Verification items for the finished model (mm, model axes). A direction names the side the tool comes from. Round coordinates to 2 decimals unless told otherwise and drop trailing zeros. Order: outer loops, then holes, each group sorted by start corner. A loop starts at its lowest first (then second) coordinate and runs counter-clockwise, first axis right, second up. Notation, with made-up numbers: (-35.5, 6) -> (-21.5, 6) arc R16 ccw to (-21.5, 37) -> close; hole circle Ø5 at (17, 32.5). An arc over 180 degrees is marked (long way). Write item = value, one per line. Start each with the question number.
from build123d import *

# Parameters (mm, degrees)
SKETCH1_W            = 208
SKETCH1_H            = 147
BOSS_EXTRUDE1_DEPTH  = 5
CUT_EXTRUDE1_DEPTH   = 129.501744983
SKETCH3_W            = 88.802487793
SKETCH3_H            = 5
CUT_EXTRUDE2_DEPTH   = 5
MIRROR3_COPY_1_DEPTH = 129.501744983
FILLET1_R            = 10
CUT_EXTRUDE3_DEPTH   = 129.501744983
BOSS_EXTRUDE2_DEPTH  = 20
FILLET2_R            = 5
FILLET2_OF_MIRROR4_R = 5
MIRROR5_START        = -20
MIRROR5_DEPTH        = 20


# Read off the part's stored shape, not the designer's step: Mirror5
with BuildPart() as part:
    # Sketch1 → Boss-Extrude1 (new body)
    with BuildSketch(Plane(origin=(0, 0, 0), x_dir=(1, 0, 0), z_dir=(0, 1, 0))):
        with Locations((0, -1.810679612)):
            Rectangle(SKETCH1_W, SKETCH1_H)
    extrude(amount=BOSS_EXTRUDE1_DEPTH)

    # Sketch2 → Cut-Extrude1 (cut, through all)
    with BuildSketch(Plane(origin=(0, 5, 0), x_dir=(1, 0, 0), z_dir=(0, 1, 0))):
        with BuildLine():
            Line((-89, 75), (-89, 55))
            Line((-89, 55), (-44, 55))
            Line((-44, 55), (-44, 50))
            Line((-44, 50), (-29, 50))
            Line((-29, 50), (-29, 53))
            Line((-29, 53), (-14, 53))
            ThreePointArc((-14, 53), (-6.928932188, 53.502525317), (0, 55))
            Line((0, 55), (0, 75))
            Line((0, 75), (-89, 75))
        make_face()
    cut_extrude1 = extrude(amount=-CUT_EXTRUDE1_DEPTH, mode=Mode.SUBTRACT)

    # Mirror1: Cut-Extrude1 across plane
    add(cut_extrude1.mirror(Plane.XY), mode=Mode.SUBTRACT)

    # Sketch3 → Cut-Extrude2 (cut)
    with BuildSketch(Plane.XY.offset(75.310679612)):
        with Locations((-44.401243897, 2.5)):
            Rectangle(SKETCH3_W, SKETCH3_H)
    cut_extrude2 = extrude(amount=-CUT_EXTRUDE2_DEPTH, mode=Mode.SUBTRACT)

    # Mirror3: Cut-Extrude1, Cut-Extrude2 across plane
    add(cut_extrude1.mirror(Plane(origin=(0, 0, 0), x_dir=(0, 0, 1), z_dir=(1, 0, 0))), mode=Mode.SUBTRACT)
    add(cut_extrude2.mirror(Plane(origin=(0, 0, 0), x_dir=(0, 0, 1), z_dir=(1, 0, 0))), mode=Mode.SUBTRACT)

    # Mirror3 copy 1 sketch → Mirror3 copy 1 (cut, through all)
    with BuildSketch(Plane(origin=(0, 5, 0), x_dir=(-1, 0, 0), z_dir=(0, 1, 0))):
        with BuildLine():
            Line((-89, 75), (-89, 55))
            Line((-89, 55), (-44, 55))
            Line((-44, 55), (-44, 50))
            Line((-44, 50), (-29, 50))
            Line((-29, 50), (-29, 53))
            Line((-29, 53), (-14, 53))
            ThreePointArc((-14, 53), (-6.928932188, 53.502525317), (0, 55))
            Line((0, 55), (0, 75))
            Line((0, 75), (-89, 75))
        make_face()
    extrude(amount=-MIRROR3_COPY_1_DEPTH, mode=Mode.SUBTRACT)

    # Fillet1
    fillet1_edges = [part.edges().sort_by_distance(p)[0] for p in [
        (104, 2.5, 75.310679612),
        (-104, 2.5, 75.310679612),
        (-104, 2.5, -71.689320388),
        (104, 2.5, -71.689320388),
    ]]
    fillet(fillet1_edges, radius=FILLET1_R)

    # Sketch4 → Cut-Extrude3 (cut, through all)
    with BuildSketch(Plane(origin=(0, 5, 0), x_dir=(1, 0, 0), z_dir=(0, 1, 0))):
        with BuildLine():
            Line((-52.239573725, -2.137194831), (-52.239573725, -12.224477428))
            ThreePointArc((-52.239573725, -12.224477428), (-52.093127116, -12.578030818), (-51.739573725, -12.724477428))
            Line((-51.739573725, -12.724477428), (-49.914138918, -12.724477428))
            ThreePointArc((-49.914138918, -12.724477428), (-49.560585528, -12.578030818), (-49.414138918, -12.224477428))
            Line((-49.414138918, -12.224477428), (-49.414138918, -2.137194831))
            ThreePointArc((-49.414138918, -2.137194831), (-49.267692309, -1.783641441), (-48.914138918, -1.637194831))
            Line((-48.914138918, -1.637194831), (-37.856129593, -1.637194831))
            ThreePointArc((-37.856129593, -1.637194831), (-37.502576202, -1.490748222), (-37.356129593, -1.137194831))
            Line((-37.356129593, -1.137194831), (-37.356129593, 0.688239976))
            ThreePointArc((-37.356129593, 0.688239976), (-37.502576202, 1.041793366), (-37.856129593, 1.188239976))
            Line((-37.856129593, 1.188239976), (-48.914138918, 1.188239976))
            ThreePointArc((-48.914138918, 1.188239976), (-49.267692309, 1.334686585), (-49.414138918, 1.688239976))
            Line((-49.414138918, 1.688239976), (-49.414138918, 11.775522572))
            ThreePointArc((-49.414138918, 11.775522572), (-49.560585528, 12.129075963), (-49.914138918, 12.275522572))
            Line((-49.914138918, 12.275522572), (-51.739573725, 12.275522572))
            ThreePointArc((-51.739573725, 12.275522572), (-52.093127116, 12.129075963), (-52.239573725, 11.775522572))
            Line((-52.239573725, 11.775522572), (-52.239573725, 1.688239976))
            ThreePointArc((-52.239573725, 1.688239976), (-52.386020335, 1.334686585), (-52.739573725, 1.188239976))
            Line((-52.739573725, 1.188239976), (-61.856129593, 1.188239976))
            ThreePointArc((-61.856129593, 1.188239976), (-62.209682983, 1.041793366), (-62.356129593, 0.688239976))
            Line((-62.356129593, 0.688239976), (-62.356129593, -1.137194831))
            ThreePointArc((-62.356129593, -1.137194831), (-62.209682983, -1.490748222), (-61.856129593, -1.637194831))
            Line((-61.856129593, -1.637194831), (-52.739573725, -1.637194831))
            ThreePointArc((-52.739573725, -1.637194831), (-52.386020335, -1.783641441), (-52.239573725, -2.137194831))
        make_face()
    extrude(amount=-CUT_EXTRUDE3_DEPTH, mode=Mode.SUBTRACT)

    # Sketch5 → Boss-Extrude2 (add)
    with BuildSketch(Plane.XZ):
        Polygon((-104, 44.093533077), (-7.462222255, 44.093533077), (-7.462222255, 53.429268089), (-4.462222255, 53.429268089), (-4.462222255, 41.093533077), (-104, 41.093533077), align=None)
    boss_extrude2 = extrude(amount=BOSS_EXTRUDE2_DEPTH)

    # Fillet2
    fillet2_edges = [part.edges().sort_by_distance(p)[0] for p in [
        (-4.462222255, -10, 41.093533077),
    ]]
    fillet(fillet2_edges, radius=FILLET2_R)

    # Mirror4: Boss-Extrude2 across plane
    add(boss_extrude2.mirror(Plane.XY))

    # Fillet2 of Mirror4
    fillet2_of_mirror4_edges = [part.edges().sort_by_distance(p)[0] for p in [
        (-4.462222255, -10, -41.093533077),
    ]]
    fillet(fillet2_of_mirror4_edges, radius=FILLET2_OF_MIRROR4_R)

    # Mirror5 outline → Mirror5 (add)
    with BuildSketch(Plane(origin=(0, 0, 0), x_dir=(1, 0, 0), z_dir=(0, 1, 0)).offset(MIRROR5_START)):
        with BuildLine():
            Line((104, -44.093533077), (104, -41.093533077))
            Line((104, -41.093533077), (9.462222255, -41.093533077))
            ThreePointArc((9.462222255, -41.093533077), (5.926688349, -42.557999171), (4.462222255, -46.093533077))
            Line((4.462222255, -46.093533077), (4.462222255, -53.429268089))
            Line((4.462222255, -53.429268089), (7.462222255, -53.429268089))
            Line((7.462222255, -53.429268089), (7.462222255, -44.093533077))
            Line((7.462222255, -44.093533077), (104, -44.093533077))
        make_face()
        with BuildLine():
            Line((9.462222255, 41.093533077), (104, 41.093533077))
            Line((104, 41.093533077), (104, 44.093533077))
            Line((104, 44.093533077), (7.462222255, 44.093533077))
            Line((7.462222255, 44.093533077), (7.462222255, 53.429268089))
            Line((7.462222255, 53.429268089), (4.462222255, 53.429268089))
            Line((4.462222255, 53.429268089), (4.462222255, 46.093533077))
            ThreePointArc((4.462222255, 46.093533077), (5.926688349, 42.557999171), (9.462222255, 41.093533077))
        make_face()
    extrude(amount=MIRROR5_DEPTH)


solid = part.part
(1) Cross-section at D-D (x = 64.5). Enter the section's corners in (y, z), and give its area (3 significant figures).
(2) Scan lines: line 1 along Z through (x, y) = (22, -4.5); line 2 along X through (y, z) = (-14, -49.5); line 3 along Z through (x, y) = (-38.5, 2.25). Record each from-to range of solid material in increasing order. Write a range as from..to.
(3) Draft check along X on faces 4 (the cylindrical face through (100.99, 2.54, -68.84)), 5 (the flat face through (-7.462, -10, -49)), 6 (the flat face through (-22, 3, 53)), 7 (the cylindrical face through (-5.966, -10.14, -42.519)). Enter one of: +X half, -X half, draft (parallel to the pull), parting line (faces both ways), or undercut.
(4) Depth check by flat-ended pin: pin 1 (5 mm diameter, centred on x = 26.5, y = -17.5, fed in from -Z); pin 2 (1.5 mm diameter, centred on x = -36.5, y = 2, fed in from +Z); pin 3 (6 mm diameter, centred on x = -3.5, z = 22.5, fed in from -Y). Enter the tip coordinate at first touch or a pass-through.
(5) Set-up check for faces 1 (the cylindrical face through (-5.966, -10.14, 42.519)), 2 (the flat face through (57, -10, 41.094)), 3 (the flat face through (22, 3, 53)): record each of +Z, -Z, +X, -X, +Y, -Y from which the full face is reachable in a straight line by a thin tool's end or side.
(6) Cross-section at A-A (y = -15.25). Enter the section's corners in (x, z), and give its area (3 significant figures).
(7) Cross-section at B-B (x = 19). Enter the section's corners in (y, z).
(8) Cross-section at C-C (z = -22). Enter the section's corners in (x, y).
Outcome:
q1.outline = (-20, -44.09) -> (0, -44.09) -> (0, -55) -> (5, -55) -> (5, 55) -> (0, 55) -> (0, 44.09) -> (-20, 44.09) -> (-20, 41.09) -> (0, 41.09) -> (0, -41.09) -> (-20, -41.09) -> close
q1.area = 670 mm^2
q2.line_1 = -44.09..-41.09, 41.09..44.09
q2.line_2 = -7.46..-4.46, 4.46..7.46
q2.line_3 = -50..-1.19, 1.64..50
q3.face_4 = +X half
q3.face_5 = -X half
q3.face_6 = undercut
q3.face_7 = undercut
q4.pin_1 = -44.09
q4.pin_2 = 50
q4.pin_3 = 0
q5.face_1 = -Y
q5.face_2 = +X, -X, -Y
q5.face_3 = +Z, +Y, -Y
q6.outline = (-104, -44.09) -> (-7.46, -44.09) -> (-7.46, -53.43) -> (-4.46, -53.43) -> (-4.46, -46.09) arc R5 ccw to (-9.46, -41.09) -> (-104, -41.09) -> close; (-104, 41.09) -> (-9.46, 41.09) arc R5 ccw to (-4.46, 46.09) -> (-4.46, 53.43) -> (-7.46, 53.43) -> (-7.46, 44.09) -> (-104, 44.09) -> close; (4.46, -53.43) -> (7.46, -53.43) -> (7.46, -44.09) -> (104, -44.09) -> (104, -41.09) -> (9.46, -41.09) arc R5 ccw to (4.46, -46.09) -> close; (4.46, 46.09) arc R5 ccw to (9.46, 41.09) -> (104, 41.09) -> (104, 44.09) -> (7.46, 44.09) -> (7.46, 53.43) -> (4.46, 53.43) -> close
q6.area = 1,290 mm^2
q7.outline = (-20, -44.09) -> (0, -44.09) -> (0, -53) -> (5, -53) -> (5, 53) -> (0, 53) -> (0, 44.09) -> (-20, 44.09) -> (-20, 41.09) -> (0, 41.09) -> (0, -41.09) -> (-20, -41.09) -> close
q8.outline = (-104, 0) -> (104, 0) -> (104, 5) -> (-104, 5) -> close
